Build history of the part. All positions in model axes, mm. A direction names the side the tool comes from. Coordinates: 2 decimals unless noted, no trailing zeros. One line per item, written item: value. Start each with the question number.
```python
from build123d import *

# Parameters (mm, degrees)
SKETCH1_W               = 127
SKETCH1_H               = 127
BOSS_EXTRUDE1_DEPTH     = 5.08
CUT_EXTRUDE1_REACH      = 7.08
SKETCH2_R               = 5.3467
SKETCH4_R               = 11.1379
SKETCH4_R_2             = 7.9121
CUT_EXTRUDE3_DEPTH      = 2.159
SKETCH6_R               = 3.96875
CUT_EXTRUDE5_DEPTH      = 5.08
CIRPATTERN2_COUNT       = 9
CUT_EXTRUDE6_REACH      = 7.08
SKETCH7_R               = 3.175
SKETCH9_R               = 19.05
SKETCH9_R_2             = 5.3467
BOSS_EXTRUDE2_DEPTH     = 1.27
SKETCH10_W              = 168.716053106
SKETCH10_H              = 169.87414825
SKETCH10_R              = 47.625
CUT_EXTRUDE7_DEPTH      = 1
CUT_EXTRUDE7_DEPTH_BACK = 7.35
SKETCH16_R              = 19.05
SKETCH16_R_2            = 10.9855
BOSS_EXTRUDE3_DEPTH     = 0.762
CHAMFER1_SIZE           = 0.508
CIRPATTERN3_COUNT       = 6


with BuildPart() as part:
    # Sketch1 → Boss-Extrude1 (new body)
    with BuildSketch(Plane(origin=(0, 0, 0), x_dir=(1, 0, 0), z_dir=(0, 1, 0))):
        Rectangle(SKETCH1_W, SKETCH1_H)
    extrude(amount=BOSS_EXTRUDE1_DEPTH)

    # Sketch2 → Cut-Extrude1 (cut, up to next)
    with BuildSketch(Plane(origin=(0, 5.08, 0), x_dir=(1, 0, 0), z_dir=(0, 1, 0)), mode=Mode.PRIVATE) as cut_extrude1_sk1:
        Circle(SKETCH2_R)
    cut_extrude1_tool1 = extrude(cut_extrude1_sk1.sketch, amount=-CUT_EXTRUDE1_REACH, mode=Mode.PRIVATE) & part.part
    add(cut_extrude1_tool1.solids().sort_by_distance((0, 5.08, 0))[0], mode=Mode.SUBTRACT)

    # Sketch4 → Cut-Extrude3 (cut)
    with BuildSketch(Plane(origin=(0, 5.08, 0), x_dir=(1, 0, 0), z_dir=(0, 1, 0))):
        Circle(SKETCH4_R)
        Circle(SKETCH4_R_2, mode=Mode.SUBTRACT)
    extrude(amount=-CUT_EXTRUDE3_DEPTH, mode=Mode.SUBTRACT)

    # Sketch6 → Cut-Extrude5 (cut)
    with BuildSketch(Plane(origin=(0, 5.08, 0), x_dir=(1, 0, 0), z_dir=(0, 1, 0))):
        with Locations((17.4625, -30.245937227)):
            Circle(SKETCH6_R)
    cut_extrude5 = extrude(amount=-CUT_EXTRUDE5_DEPTH, mode=Mode.SUBTRACT)

    # CirPattern2: Cut-Extrude5 ×9 about axis
    cirpattern2_axis = Axis((0, 0, 0), (0, 1, 0))
    for i in range(1, CIRPATTERN2_COUNT):
        add(cut_extrude5.rotate(cirpattern2_axis, i * 360 / CIRPATTERN2_COUNT), mode=Mode.SUBTRACT)

    # Sketch7 → Cut-Extrude6 (cut, up to next)
    with BuildSketch(Plane(origin=(0, 5.08, 0), x_dir=(1, 0, 0), z_dir=(0, 1, 0)), mode=Mode.PRIVATE) as cut_extrude6_sk1:
        with Locations((57.15, 57.15)):
            Circle(SKETCH7_R)
    cut_extrude6_tool1 = extrude(cut_extrude6_sk1.sketch, amount=-CUT_EXTRUDE6_REACH, mode=Mode.PRIVATE) & part.part
    add(cut_extrude6_tool1.solids().sort_by_distance((57.15, 5.08, -57.15))[0], mode=Mode.SUBTRACT)
    # Sketch7 → Cut-Extrude6 (cut, up to next)
    with BuildSketch(Plane(origin=(0, 5.08, 0), x_dir=(1, 0, 0), z_dir=(0, 1, 0)), mode=Mode.PRIVATE) as cut_extrude6_sk2:
        with Locations((57.15, -57.15)):
            Circle(SKETCH7_R)
    cut_extrude6_tool2 = extrude(cut_extrude6_sk2.sketch, amount=-CUT_EXTRUDE6_REACH, mode=Mode.PRIVATE) & part.part
    add(cut_extrude6_tool2.solids().sort_by_distance((57.15, 5.08, 57.15))[0], mode=Mode.SUBTRACT)
    # Sketch7 → Cut-Extrude6 (cut, up to next)
    with BuildSketch(Plane(origin=(0, 5.08, 0), x_dir=(1, 0, 0), z_dir=(0, 1, 0)), mode=Mode.PRIVATE) as cut_extrude6_sk3:
        with Locations((-57.15, -57.15)):
            Circle(SKETCH7_R)
    cut_extrude6_tool3 = extrude(cut_extrude6_sk3.sketch, amount=-CUT_EXTRUDE6_REACH, mode=Mode.PRIVATE) & part.part
    add(cut_extrude6_tool3.solids().sort_by_distance((-57.15, 5.08, 57.15))[0], mode=Mode.SUBTRACT)
    # Sketch7 → Cut-Extrude6 (cut, up to next)
    with BuildSketch(Plane(origin=(0, 5.08, 0), x_dir=(1, 0, 0), z_dir=(0, 1, 0)), mode=Mode.PRIVATE) as cut_extrude6_sk4:
        with Locations((-57.15, 57.15)):
            Circle(SKETCH7_R)
    cut_extrude6_tool4 = extrude(cut_extrude6_sk4.sketch, amount=-CUT_EXTRUDE6_REACH, mode=Mode.PRIVATE) & part.part
    add(cut_extrude6_tool4.solids().sort_by_distance((-57.15, 5.08, -57.15))[0], mode=Mode.SUBTRACT)

    # Sketch9 → Boss-Extrude2 (add)
    with BuildSketch(Plane.XZ):
        Circle(SKETCH9_R)
        Circle(SKETCH9_R_2, mode=Mode.SUBTRACT)
    extrude(amount=BOSS_EXTRUDE2_DEPTH)

    # Sketch10 → Cut-Extrude7 (cut, two sides)
    with BuildSketch(Plane(origin=(0, 5.08, 0), x_dir=(1, 0, 0), z_dir=(0, 1, 0))) as cut_extrude7_sk:
        Rectangle(SKETCH10_W, SKETCH10_H)
        Circle(SKETCH10_R, mode=Mode.SUBTRACT)
    extrude(amount=CUT_EXTRUDE7_DEPTH, mode=Mode.SUBTRACT)
    extrude(cut_extrude7_sk.sketch, amount=-CUT_EXTRUDE7_DEPTH_BACK, mode=Mode.SUBTRACT)

    # Sketch15 → Tapped Hole for #4-40 Helicoil3 (revolve, cut)
    with BuildSketch(Plane(origin=(0, 5.08, -15.24), x_dir=(0, 0, 1), z_dir=(1, 0, 0))):
        Polygon((0, 0), (0, 6.249711583), (1.524, 5.334), (1.524, 0.219970453), (1.905, 0), align=None)
    tapped_hole_for_4_40_helicoil3 = revolve(axis=Axis((0, 11.43, -15.24), (0, -1, 0)), mode=Mode.SUBTRACT)

    # Sketch16 → Boss-Extrude3 (add)
    with BuildSketch(Plane.XZ.offset(1.27)):
        Circle(SKETCH16_R)
        Circle(SKETCH16_R_2, mode=Mode.SUBTRACT)
    extrude(amount=BOSS_EXTRUDE3_DEPTH)

    # Chamfer1
    chamfer1_edges = [part.edges().sort_by_distance(p)[0] for p in [
        (-19.05, -2.032, 0),
        (-5.3467, 5.08, 0),
        (-47.625, 0, 0),
    ]]
    chamfer(chamfer1_edges, length=CHAMFER1_SIZE)

    # CirPattern3: Tapped Hole for #4-40 Helicoil3 ×6 about axis
    cirpattern3_axis = Axis((0, 0, 0), (0, 1, 0))
    for i in range(1, CIRPATTERN3_COUNT):
        add(tapped_hole_for_4_40_helicoil3.rotate(cirpattern3_axis, i * 360 / CIRPATTERN3_COUNT), mode=Mode.SUBTRACT)


solid = part.part
```
Item 1: Band-saw the part on A-A, the plane z = 0. Count the separate pieces of the cut face and the enclosed holes in it, and give its area (3 significant figures).
Item 2: Drop flat-ended pins along their axis: pin 1 Ø2 at (y, z) = (1.5, 24.5) entering from -X; pin 2 Ø9 at (x, z) = (32.82, -11.95) entering from -Y; pin 3 Ø3 at (y, z) = (-1, 30) entering from -X. Give the stop position or say it passes through.
Item 3: Two-plate mould, pull along Z, no slides. Class faces 4 (the face through (-11.3, 5.08, -0.7)), 5 (the face through (-37.794, 2.826, 28.979)), 6 (the face through (31.96, 2.58, -8.07)): +Z half, -Z half, draft (parallel to the pull), parting line (faces both ways), or undercut.
Item 4: Tool access for faces 1 (the face through (5, -1.27, 3)), 2 (the face through (-27.271, 2.576, -26.384)), 3 (the face through (11.687, 2.339, 7.422)): list every direction of +Z, -Z, +X, -X, +Y, -Y with a clear straight run to the whole face (end or side of a thin tool).
Item 5: Probe probe 1 along X at (y, z) = (1.1, -7.62); probe 2 along X at (y, z) = (3.25, -9.5); probe 3 along Y at (x, z) = (2, 24). List the from-to ranges inside material, lowest first.
Worked out:
1. separate pieces: 3
1. enclosed holes: 0
1. area: 422 mm²
2. pin 1: stops at x = -41.42
2. pin 2: stops at y = 0
2. pin 3: stops at x = -37.32
3. face 4: draft
3. face 5: parting line
3. face 6: undercut
4. face 1: -Y
4. face 2: +Y, -Y
4. face 3: +Y
5. probe 1: x = -47.01 to -14.72, -11.67 to 11.67, 14.72 to 47.01
5. probe 2: x = -46.67 to -5.81, 5.81 to 29.69, 35.94 to 46.67
5. probe 3: y = 0 to 5.08
